Input: part model. Units: mm. Frame: model coordinates. A direction names the side the tool comes from. Coordinates: 2 decimals unless noted, no trailing zeros. Write each loop counter-clockwise with the first axis right and the second up, starting at its lowest first coordinate (ties: lowest second). Pieces come first, ordered by that corner, then holes. Notation, with made-up numbers: M 55.25,33 L 86.25,33 A30 ccw 86.25,72 Z; hole C -19,9 d11. An arc over 180 degrees is marked long. Write each question's results on one line, items separated by ' | '. Start each with the question number.
1. Set-up query: faces 1 (the flat face through (1, -3.5, 0)), 2 (the cylindrical face through (21.51, 0.63, -0.04)), 3 (the flat face through (0, 3.5, 0)), 4 (the cylindrical face through (-23.2, 2.4, 3.4)). Return all of +Z, -Z, +X, -X, +Y, -Y with unobstructed straight access to the full face (end or side cutting, diameter ignored); none if empty.
2. First-contact query: pin 1 (5.5 mm diameter, centred on x = 0.5, z = 0, fed in from -Y); pin 2 (3 mm diameter, centred on x = -20, y = 0, fed in from +Z); pin 3 (1 mm diameter, centred on y = 1.5, z = 2.5, fed in from -X); pin 4 (4 mm diameter, centred on x = 1, z = 1, fed in from +Y). Flat tips, straight axial feed; report the tip coordinate or a pass-through.
3. Ray query, probe 1 along Y at (x, z) = (-20, 6) (3 decimals); probe 2 along Z at (x, y) = (11.5, -2); probe 3 along Y at (x, z) = (13, 0.5). Return the intervals inside material, ascending.
4. Section query C-C, the plane y = 0. Output: boundary loops of the cut face in (x, z) (3 decimals).
5. Section query A-A, the plane z = 0.75. Output: boundary loops of the cut face in (x, y) (1 decimal).
6. Section query D-D, the plane z = 8.5. Output: boundary loops of the cut face in (x, y) (3 decimals).
7. Section query B-B, the plane x = -20. Output: boundary loops of the cut face in (y, z) (3 decimals), and give its area (3 significant figures).
Autodesk Inventor part; units mm, degrees
ref_plane "YZ Plane" through (0, 0, 0) normal (1, 0, 0) x (0, 1, 0)
ref_plane "XZ Plane" through (0, 0, 0) normal (0, 1, 0) x (-1, 0, 0)
ref_plane "XY Plane" through (0, 0, 0) normal (0, 0, 1) x (1, 0, 0)
sketch "スケッチ1" plane through (0, 0, 0) normal (0, 0, 1) x (1, 0, 0)
  line L0 (-22.5, 3.5) -> (22.5, 3.5)
  line L1 (22.5, 3.5) -> (22.5, -3.5)
  line L2 (22.5, -3.5) -> (-22.5, -3.5)
  line L3 (-22.5, -3.5) -> (-22.5, 3.5)
  line L4 (-22.5, 3.5) -> (22.5, -3.5) construction
  line L5 (22.5, 3.5) -> (-22.5, -3.5) construction
  line L6 (0, -11.2) -> (0, 11.2) construction
  line L7 (-38.51, 0) -> (35.06, 0) construction
  circle A0 centre (-20, 0) radius 4.55
  line L8 (22.5, -3.5) -> (22.5, 3.5)
  circle A1 centre (20, 0) radius 4.55
  circle A2 centre (20, 0) radius 1.635
  circle A3 centre (-20, 0) radius 1.635
  circle A4 centre (-20, 0) radius 4
  line L9 (-20, 4) -> (-20, -4) construction
  circle A5 centre (-20, 6) radius 2
  circle A6 centre (-20, -6) radius 2
  circle A7 centre (-20, 0) radius 4
  circle A8 centre (-20, 0) radius 8
  point P0 (0, 0)
  point P1 (-17.0927, 3.5)
  point P2 (-22.9073, 3.5)
  point P3 (-22.9073, -3.5)
  point P4 (-17.0927, -3.5)
  point P5 (17.0927, 3.5)
  point P6 (17.0927, -3.5)
  point P7 (22.9073, -3.5)
  point P8 (22.9073, 3.5)
  dimension "d1" = 7
  dimension "d2" = 20
  dimension "d3" = 45
  dimension "d4" = 9.1
  dimension "d13" = 3.27
  dimension "d14" = 3.27
  dimension "d15" = 8
  dimension "d16" = 4
  dimension "d17" = 4
  dimension "d18" = 12
extrude "押し出し1" add sketch "スケッチ1" along normal mid plane 5 contours L0 A4 L3 | L0 A4 L2 L3 | L0 A0 L2 A4 | A4 L2 L3 | L0 A8 L2 A0 | L0 A1 L2 A8 | L0 L1 L2 A1 picked at (19.7985, -2.8744)
fillet "フィレット1" radius 3 4 edges at (-22.5, 3.5, 0) (-22.5, -3.5, 0) (22.5, -3.5, 0) (22.5, 3.5, 0)
extrude "押し出し3" add sketch "スケッチ1" along normal blind 12 from surface at -2.5 contours A4 L0 | L0 A4 L2 L3 | L3 A4 | L2 A4
properties part number "link_arm_1"
Answer:
1) face 1: +Z, -Z, +X, -Y | face 2: +Z, -Z | face 3: +Z, -Z, +X, +Y | face 4: +Z
2) pin 1: y = -3.5 | pin 2: through | pin 3: x = -23.87 | pin 4: y = 3.5
3) probe 1: -4 to -1.635, 1.635 to 4 | probe 2: -2.5 to 2.5 | probe 3: -3.5 to 3.5
4) outline: M -24,-2.5 L -21.635,-2.5 L -21.635,9.5 L -24,9.5 Z; M -18.365,-2.5 L 18.365,-2.5 L 18.365,2.5 L -16,2.5 L -16,9.5 L -18.365,9.5 Z; M 21.635,-2.5 L 22.5,-2.5 L 22.5,2.5 L 21.635,2.5 Z
5) outline: M -18.1,-3.5 L 19.5,-3.5 A3 ccw 22.5,-0.5 L 22.5,0.5 A3 ccw 19.5,3.5 L -18.1,3.5 A4 ccw long Z; hole C -20,0 d3.3; hole C 20,0 d3.3
6) outline: C -20,0 d8; hole C -20,0 d3.27
7) outline: M -4,-2.5 L -1.635,-2.5 L -1.635,9.5 L -4,9.5 Z; M 1.635,-2.5 L 4,-2.5 L 4,9.5 L 1.635,9.5 Z | area: 56.8 mm^2
